```python
from build123d import *

# Parameters (mm, degrees)
SKETCH2_R           = 19.05
SKETCH2_W           = 6.858
SKETCH2_H           = 6.858
BOSS_EXTRUDE1_DEPTH = 63.5
BOSS_EXTRUDE2_DEPTH = 63.5
CIRPATTERN1_COUNT   = 8


with BuildPart() as part:
    # Sketch2 → Boss-Extrude1 (new body)
    with BuildSketch(Plane(origin=(0, 0, 0), x_dir=(1, 0, 0), z_dir=(0, 1, 0))):
        with Locations(Location((0, 0, 0), (0, 0, 270))):
            Circle(SKETCH2_R)
        Rectangle(SKETCH2_W, SKETCH2_H, mode=Mode.SUBTRACT)
    extrude(amount=BOSS_EXTRUDE1_DEPTH)

    # Sketch3 → Boss-Extrude2 (add)
    with BuildSketch(Plane(origin=(0, 0, 0), x_dir=(1, 0, 0), z_dir=(0, 1, 0))):
        with BuildLine():
            Line((0, 22.86), (0, 19.05))
            ThreePointArc((0, 19.05), (1.272844406, 19.007429261), (2.54, 18.879907309))
            Line((2.54, 18.879907309), (7.283289763, 22.86))
            Line((7.283289763, 22.86), (0, 22.86))
        make_face()
        with BuildLine():
            ThreePointArc((-2.54, 18.879907309), (-1.272844406, 19.007429261), (0, 19.05))
            Line((0, 19.05), (0, 22.86))
            Line((0, 22.86), (-7.283289763, 22.86))
            Line((-7.283289763, 22.86), (-2.54, 18.879907309))
        make_face()
    boss_extrude2 = extrude(amount=BOSS_EXTRUDE2_DEPTH)

    # CirPattern1: Boss-Extrude2 ×8 about axis
    cirpattern1_axis = Axis((0, 0, 0), (0, 1, 0))
    for i in range(1, CIRPATTERN1_COUNT):
        add(boss_extrude2.rotate(cirpattern1_axis, i * 360 / CIRPATTERN1_COUNT))


solid = part.part
```
The model under review builds one solid part; all positions refer to its coordinate system, in mm. A direction names the side the tool comes from. Coordinates: 2 decimals unless noted, no trailing zeros. Write each loop counter-clockwise with the first axis right and the second up, starting at its lowest first coordinate (ties: lowest second). Pieces come first, ordered by that corner, then holes. Notation, with made-up numbers: (1, 67.25) -> (52, 67.25) arc R12 cw to (52, 83.25) -> close; hole circle Ø7 at (-37, -37.5). An arc over 180 degrees is marked (long way). One line per item, written item: value. Start each with the question number.
Q1. Add section C-C, the plane z = -5. Give the boundary of the cut face in (x, y), then the cut area to 3 significant figures.
Q2. Add section A-A, the plane x = -0.5. Give the boundary of the cut face in (y, z).
Q3. For faces 1 (the face through (-16.24, 31.31, 16.09)), 2 (the face through (-3.429, 31, 0)), list the 3-axis set-ups (+Z, -Z, +X, -X, +Y, -Y) from which the entire face can be reached by the end or side of a thin tool; tool diameter is ignored.
Q4. Add section B-B, the plane z = 0. Give the boundary of the cut face in (x, y), then the cut area to 3 significant figures.
Q5. Add section D-D, the plane x = -20. Give the boundary of the cut face in (y, z), then the cut area to 3 significant figures.
Q6. The part is to be moulded in two halves that separate along Z. For faces 3 (the face through (-7.354, 31.306, 17.573)), 4 (the face through (0, 31, -22.86)), 5 (the face through (0, 31, 22.86)), 6 (the face through (4.878, 31.306, -20.842)), say which applies: +Z half, -Z half, draft (parallel to the pull), parting line (faces both ways), or undercut.
Q7. To check wall thickness, follow probe 1 along Z at (x, y) = (16.5, 22); probe 2 along Z at (x, y) = (0.5, 54). State the ranges of each line that lie inside material, in increasing order.
Q8. Clearance check with flat-ended pins moving along their axes: P1, Ø1.5, axis at x = 13.5, y = 8, coming from the -Z side; P2, Ø3, axis at x = 11, y = 28.5, coming from the -Z side. State where each tip first meets the part, or that it passes through.
Response:
1. outline: (-22.86, 0) -> (-20.94, 0) -> (-20.94, 63.5) -> (-22.86, 63.5) -> close; (-18.38, 0) -> (18.38, 0) -> (18.38, 63.5) -> (-18.38, 63.5) -> close; (20.94, 0) -> (22.86, 0) -> (22.86, 63.5) -> (20.94, 63.5) -> close
1. area: 2,580 mm²
2. outline: (0, -22.86) -> (63.5, -22.86) -> (63.5, -3.43) -> (0, -3.43) -> close; (0, 3.43) -> (63.5, 3.43) -> (63.5, 22.86) -> (0, 22.86) -> close
3. face 1: +Z, -X, +Y, -Y
3. face 2: +Y, -Y
4. outline: (-22.86, 0) -> (-3.43, 0) -> (-3.43, 63.5) -> (-22.86, 63.5) -> close; (3.43, 0) -> (22.86, 0) -> (22.86, 63.5) -> (3.43, 63.5) -> close
4. area: 2,470 mm²
5. outline: (0, -12.33) -> (63.5, -12.33) -> (63.5, -11.13) -> (0, -11.13) -> close; (0, -3.87) -> (63.5, -3.87) -> (63.5, 3.87) -> (0, 3.87) -> close; (0, 11.13) -> (63.5, 11.13) -> (63.5, 12.33) -> (0, 12.33) -> close
5. area: 644 mm²
6. face 3: undercut
6. face 4: -Z half
6. face 5: +Z half
6. face 6: undercut
7. probe 1: -15.83 to -11.44, -9.52 to 9.52, 11.44 to 15.83
7. probe 2: -22.86 to -3.43, 3.43 to 22.86
8. P1: z = -19.58
8. P2: z = -21.31
